Input: part model. Units: mm. Frame: model coordinates. Face numbers are marked on the shaded views. Coordinates: 2 decimals unless noted, no trailing zeros. Write each loop counter-clockwise with the first axis right and the second up, starting at its lowest first coordinate (ties: lowest second). Pieces come first, ordered by that corner, then holes.
1) Section query D-D (y = 20.75). Output: boundary loops of the cut face in (x, z).
2) Section query A-A (x = -17.5). Output: boundary loops of the cut face in (y, z).
3) Draft query along Z for the marked faces 1, 2, 3 and 4. Return one class per face: pulls with the +Z half, pulls with the -Z half, needs draft (parallel to the pull), parting line crosses it, or undercut.
4) Line query: L1, parallel to Y at x = 0, z = -26.5; L2, parallel to Z at x = -17.5, y = 3.25; L3, parallel to Z at x = -5, y = 13.75. Output: solid intervals per line, ascending.
5) Pin query (flat end, axial travel): pin 1 Ø8 at (x, z) = (20.5, -20.5) entering from -Y; pin 2 Ø8 at (x, z) = (-11.5, 6) entering from +Y; pin 3 Ø5 at (y, z) = (18, -23) entering from +X. Return the tip coordinate at first contact, or that it passes through.
6) Section query C-C (z = 0). Output: boundary loops of the cut face in (x, y), then the cut area to 3 significant figures.
7) Section query B-B (x = 0). Output: boundary loops of the cut face in (y, z).
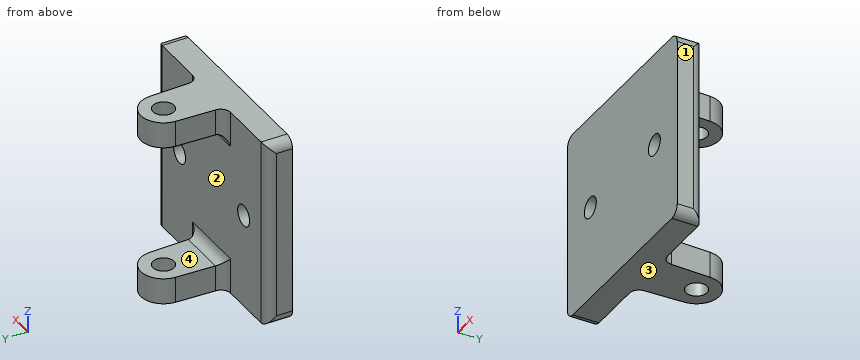
from build123d import *

# Parameters (mm, degrees)
SKETCH2_W           = 60
SKETCH2_H           = 58
SKETCH2_R           = 3.25
BOSS_EXTRUDE1_DEPTH = 8
SKETCH3_R           = 3.25
BOSS_EXTRUDE2_DEPTH = 8
FILLET1_R           = 3


with BuildPart() as part:
    # Sketch2 → Boss-Extrude1 (new body)
    with BuildSketch(Plane(origin=(0, 0, 0), x_dir=(1, 0, 0), z_dir=(0, 1, 0))):
        Rectangle(SKETCH2_W, SKETCH2_H)
        with Locations((-17.5, 0)):
            Circle(SKETCH2_R, mode=Mode.SUBTRACT)
        with Locations((17.5, 0)):
            Circle(SKETCH2_R, mode=Mode.SUBTRACT)
    extrude(amount=BOSS_EXTRUDE1_DEPTH)

    # Sketch3 → Boss-Extrude2 (add)
    with BuildSketch(Plane.XY.offset(29)):
        with BuildLine():
            Line((-7.5, 8), (-6.996052809, 23))
            ThreePointArc((-6.996052809, 23), (0, 29.764957256), (6.996052809, 23))
            Line((6.996052809, 23), (7.5, 8))
            Line((7.5, 8), (-7.5, 8))
        make_face()
        with Locations((0, 22.764957256)):
            Circle(SKETCH3_R, mode=Mode.SUBTRACT)
    boss_extrude2 = extrude(amount=-BOSS_EXTRUDE2_DEPTH)

    # Mirror1: Boss-Extrude2 across plane
    add(boss_extrude2.mirror(Plane.XY))

    # Fillet1
    fillet1_edges = [part.edges().sort_by_distance(p)[0] for p in [
        (-30, 8, 0),
        (0, 8, 21),
        (7.5, 8, 25),
        (-7.5, 8, 25),
        (0, 8, -21),
        (-7.5, 8, -25),
        (7.5, 8, -25),
        (30, 8, 0),
        (30, 4, 29),
        (-30, 4, 29),
        (-30, 4, -29),
        (30, 4, -29),
    ]]
    fillet(fillet1_edges, radius=FILLET1_R)


solid = part.part
Answer:
1. outline: (-7.07, -29) - (-2.55, -29) - (-2.55, -21) - (-7.07, -21) - close; (-7.07, 21) - (-2.55, 21) - (-2.55, 29) - (-7.07, 29) - close; (2.55, -29) - (7.07, -29) - (7.07, -21) - (2.55, -21) - close; (2.55, 21) - (7.07, 21) - (7.07, 29) - (2.55, 29) - close
2. outline: (0, -29) - (8, -29) - (8, -3.25) - (0, -3.25) - close; (0, 3.25) - (8, 3.25) - (8, 29) - (0, 29) - close
3. face 1: needs draft
3. face 2: undercut
3. face 3: pulls with the -Z half
3. face 4: undercut
4. L1: y = 0 to 19.51, 26.01 to 29.76
4. L2: z = -29 to -3.25, 3.25 to 29
4. L3: z = -29 to -21, 21 to 29
5. pin 1: stops at y = 0
5. pin 2: stops at y = 8
5. pin 3: stops at x = 7.25
6. outline: (-30, 0) - (-20.75, 0) - (-20.75, 8) - (-27, 8) arc R3 ccw to (-30, 5) - close; (-14.25, 0) - (14.25, 0) - (14.25, 8) - (-14.25, 8) - close; (20.75, 0) - (30, 0) - (30, 5) arc R3 ccw to (27, 8) - (20.75, 8) - close
6. area: 372 mm2
7. outline: (0, -29) - (19.51, -29) - (19.51, -21) - (11, -21) arc R3 cw to (8, -18) - (8, 18) arc R3 cw to (11, 21) - (19.51, 21) - (19.51, 29) - (0, 29) - close; (26.01, -29) - (29.76, -29) - (29.76, -21) - (26.01, -21) - close; (26.01, 21) - (29.76, 21) - (29.76, 29) - (26.01, 29) - close
